Design review of the part built by this model. Coordinates are the model's own, in mm. Face numbers are marked on the shaded views. Give positions to 0.01 mm unless a question says otherwise; leave off trailing zeros. Loops run counter-clockwise (first coordinate to the right, second up) from the corner with the lowest first, then second, coordinate; pieces in that order, holes last. Notation, with made-up numbers: M 88.5,0.5 L 129.5,0.5 A24 ccw 129.5,38.5 Z; hole C 41.25,-25 d6. An arc over 180 degrees is marked long. Use a Markdown table: item, result. Add a question column.
(1) Add section D-D, the plane y = 3.75. Give the boundary of the cut face in (x, z).
(2) Add section C-C, the plane x = 0. Give the boundary of the cut face in (y, z).
(3) Draft analysis for pull direction X (two halves, no side actions). For the marked faces 1, 2 and 3, state which applies: pulls with the +X half, pulls with the -X half, needs draft (parallel to the pull), parting line crosses it, or undercut.
(4) Add section B-B, the plane z = -3.5. Give the boundary of the cut face in (x, y), then the cut area to 3 significant figures.
(5) Add section A-A, the plane y = 0. Give the boundary of the cut face in (x, z), then the cut area to 3 significant figures.
(6) For probe 1 along X at (y, z) = (2.5, 0); probe 2 along X at (y, z) = (-1.5, -3.5); probe 3 along Z at (x, y) = (0, -1.25), list the stretches that pass through material, from the lowest coordinate up.
(7) Insertion check: pin 1 Ø4.5 at (x, z) = (0, -3.5) entering from +Y; pin 2 Ø5 at (y, z) = (0, 20) entering from +X. Each pin has a flat end and moves straight along its axis. Give the tip position at first contact, or say it passes through.
```python
from build123d import *

# Parameters (mm, degrees)
ESQUISSE1_W                  = 12.5
ESQUISSE1_H                  = 12.5
BOSS_EXTRU_1_DEPTH           = 27.5
ENL_V_MAT_EXTRU_1_DEPTH      = 29.885550021
ENL_V_MAT_EXTRU_1_DEPTH_BACK = 29.885550021
ESQUISSE2_R                  = 2.85
ENL_V_MAT_EXTRU_2_DEPTH      = 29.885550021
ENL_V_MAT_EXTRU_2_DEPTH_BACK = 29.885550021
ESQUISSE3_R                  = 1.6
ENL_V_MAT_EXTRU_3_DEPTH      = 29.885550021
ENL_V_MAT_EXTRU_3_DEPTH_BACK = 29.885550021
ESQUISSE4_R                  = 2.1


with BuildPart() as part:
    # Esquisse1 → Boss.-Extru.1 (new, symmetric)
    with BuildSketch(Plane.XY):
        Rectangle(ESQUISSE1_W, ESQUISSE1_H)
    extrude(amount=BOSS_EXTRU_1_DEPTH, both=True)

    # Esquisse2 → Enlèv. mat.-Extru.1 (cut, two sides: drawn at the far end of the back side and taken through both)
    with BuildSketch(Plane(origin=(0, 0, 0), x_dir=(1, 0, 0), z_dir=(0, 1, 0)).offset(-ENL_V_MAT_EXTRU_1_DEPTH_BACK)):
        with Locations(Location((0, 3.5, 0), (0, 0, 270))):
            Circle(ESQUISSE2_R)
        with Locations(Location((0, -3.5, 0), (0, 0, 270))):
            Circle(ESQUISSE2_R)
    extrude(amount=ENL_V_MAT_EXTRU_1_DEPTH + ENL_V_MAT_EXTRU_1_DEPTH_BACK, mode=Mode.SUBTRACT)

    # Esquisse3 → Enlèv. mat.-Extru.2 (cut, two sides: drawn at the far end of the back side and taken through both)
    with BuildSketch(Plane(origin=(0, 0, 0), x_dir=(1, 0, 0), z_dir=(0, 1, 0)).offset(-ENL_V_MAT_EXTRU_2_DEPTH_BACK)):
        Circle(ESQUISSE3_R)
    extrude(amount=ENL_V_MAT_EXTRU_2_DEPTH + ENL_V_MAT_EXTRU_2_DEPTH_BACK, mode=Mode.SUBTRACT)

    # Esquisse4 → Enlèv. mat.-Extru.3 (cut, two sides: drawn at the far end of the back side and taken through both)
    with BuildSketch(Plane(origin=(0, 0, 0), x_dir=(0, 0, -1), z_dir=(1, 0, 0)).offset(-ENL_V_MAT_EXTRU_3_DEPTH_BACK)):
        with Locations((-20, 0)):
            Circle(ESQUISSE4_R)
        with Locations((20, 0)):
            Circle(ESQUISSE4_R)
    extrude(amount=ENL_V_MAT_EXTRU_3_DEPTH + ENL_V_MAT_EXTRU_3_DEPTH_BACK, mode=Mode.SUBTRACT)


solid = part.part
```
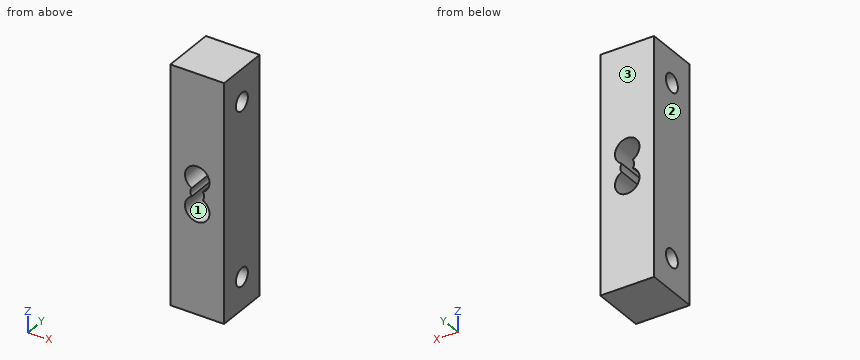
Established:
| question | item | result |
|---|---|---|
| 1 | outline | M -6.25,-27.5 L 6.25,-27.5 L 6.25,27.5 L -6.25,27.5 Z; hole M -1.28,-0.96 A2.85 ccw long 1.28,-0.96 A1.6 ccw 1.28,0.96 A2.85 ccw long -1.28,0.96 A1.6 ccw Z |
| 2 | outline | M -6.25,-27.5 L 6.25,-27.5 L 6.25,-6.35 L -6.25,-6.35 Z; M -6.25,6.35 L 6.25,6.35 L 6.25,27.5 L -6.25,27.5 Z; hole C 0,-20 d4.2; hole C 0,20 d4.2 |
| 3 | face 1 | undercut |
| 3 | face 2 | pulls with the -X half |
| 3 | face 3 | needs draft |
| 4 | outline | M -6.25,-6.25 L -2.85,-6.25 L -2.85,6.25 L -6.25,6.25 Z; M 2.85,-6.25 L 6.25,-6.25 L 6.25,6.25 L 2.85,6.25 Z |
| 4 | area | 85.0 mm^2 |
| 5 | outline | M -6.25,-27.5 L 6.25,-27.5 L 6.25,-22.1 L -6.25,-22.1 Z; M -6.25,-17.9 L 6.25,-17.9 L 6.25,17.9 L -6.25,17.9 Z; M -6.25,22.1 L 6.25,22.1 L 6.25,27.5 L -6.25,27.5 Z; hole M -1.28,-0.96 A2.85 ccw long 1.28,-0.96 A1.6 ccw 1.28,0.96 A2.85 ccw long -1.28,0.96 A1.6 ccw Z |
| 5 | area | 527 mm^2 |
| 6 | probe 1 | -6.25 to -1.6, 1.6 to 6.25 |
| 6 | probe 2 | -6.25 to -2.85, 2.85 to 6.25 |
| 6 | probe 3 | -27.5 to -21.69, -18.31 to -6.35, 6.35 to 18.31, 21.69 to 27.5 |
| 7 | pin 1 | through |
| 7 | pin 2 | x = 6.25 |
